from build123d import *

# Parameters (mm, degrees)
F0_W     = 40.64
F0_H     = 116.84
F1_DEPTH = 6.35
F0_W_2   = 50.8
F0_H_2   = 127
F2_DEPTH = 12.7
F3_R     = 3.175
F4_DEPTH = 38.1


with BuildPart() as f1:
    # F0 (on Front) → F1 (new body)
    with BuildSketch(Plane.XZ):
        Rectangle(F0_W, F0_H)
    extrude(amount=F1_DEPTH)

    # F0 (on Front) → F2 (join)
    with BuildSketch(Plane.XZ):
        Rectangle(F0_W_2, F0_H_2)
        Rectangle(F0_W, F0_H, mode=Mode.SUBTRACT)
    extrude(amount=F2_DEPTH)

    # F3 (on face) → F4 (join)
    with BuildSketch(Plane.XZ):
        with Locations((-13.335, -51.435)):
            Circle(F3_R)
        with Locations((13.335, -51.435)):
            Circle(F3_R)
        with Locations((13.335, 51.435)):
            Circle(F3_R)
        with Locations((-13.335, 51.435)):
            Circle(F3_R)
    extrude(amount=-F4_DEPTH)


solid = f1.part
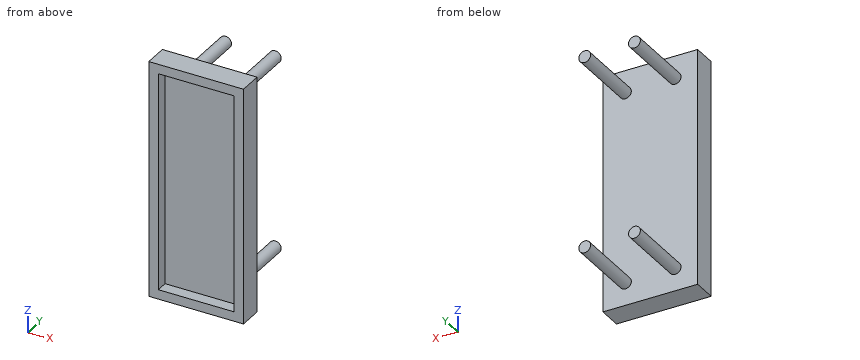
Geometry check sheet. Reference: the model listing, model coordinates, mm. Round coordinates to 2 decimals unless told otherwise and drop trailing zeros. Order: outer loops, then holes, each group sorted by start corner. A loop starts at its lowest first (then second) coordinate and runs counter-clockwise, first axis right, second up. Notation, with made-up numbers: (-26, 47.25) -> (-7, 47.25) arc R21 cw to (-7, 53.25) -> close; hole circle Ø3 at (-10, 50). An arc over 180 degrees is marked (long way). Use one line per item in the form item = value.
1. Cross-section at C-C, the plane y = 21.5. Enter the section's corners in (x, z) (3 decimals), plus the area to 3 significant figures.
Working result:
outline = circle Ø6.35 at (-13.335, -51.435); circle Ø6.35 at (-13.335, 51.435); circle Ø6.35 at (13.335, -51.435); circle Ø6.35 at (13.335, 51.435)
area = 127 mm^2
2. Go/stop test with flat-tipped pins: pin 1 (5 mm diameter, centred on x = 5.5, z = -9.5, fed in from +Y); pin 2 (1 mm diameter, centred on x = 12.5, z = 50, fed in from -Y); pin 3 (1 mm diameter, centred on x = 19, y = 3, fed in from -Z). Record where each tip stops, or that it passes through.
Working result:
pin_1 = 0
pin_2 = -6.35
pin_3 = through
3. Cross-section at D-D, the plane x = -22. Enter the section's corners in (y, z), plus the area to 3 significant figures.
Working result:
outline = (-12.7, -63.5) -> (0, -63.5) -> (0, 63.5) -> (-12.7, 63.5) -> close
area = 1,610 mm^2
4. Cross-section at B-B, the plane z = 4.5. Enter the section's corners in (x, y).
Working result:
outline = (-25.4, -12.7) -> (-20.32, -12.7) -> (-20.32, -6.35) -> (20.32, -6.35) -> (20.32, -12.7) -> (25.4, -12.7) -> (25.4, 0) -> (-25.4, 0) -> close
5. Scan lines: line 1 along X through (y, z) = (-7.5, -57.5); line 2 along Z through (x, y) = (19.5, -8.5); line 3 along Y through (x, z) = (7.5, -47). Record each from-to range of solid material in increasing order. Write a range as from..to.
Working result:
line_1 = -25.4..-20.32, 20.32..25.4
line_2 = -63.5..-58.42, 58.42..63.5
line_3 = -6.35..0
6. Cross-section at A-A, the plane x = 1. Enter the section's corners in (y, z).
Working result:
outline = (-12.7, -63.5) -> (0, -63.5) -> (0, 63.5) -> (-12.7, 63.5) -> (-12.7, 58.42) -> (-6.35, 58.42) -> (-6.35, -58.42) -> (-12.7, -58.42) -> close
